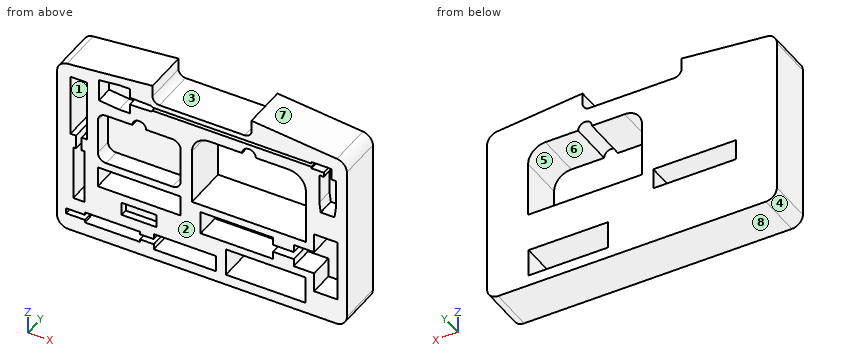
from build123d import *

# Parameters (mm, degrees)
F1_DEPTH  = 65
F11_DEPTH = 65.001
F12_DEPTH = 25.4
F13_DEPTH = 35.56
F9_W      = 120
F9_H      = 30
F8_W      = 115
F8_H      = 40
F14_DEPTH = 65.001
F15_DEPTH = 25.4
F16_DEPTH = 40.64
F10_W     = 50.8
F10_H     = 19.05
F17_DEPTH = 10.16


# Not quite as in the source:
# - a length typed as a fraction of an inch, garbled in the dataset ("3 / 203.2 mm" for 3/8 in), is restored


with BuildPart() as f1:
    # F0 (on Front) → F1 (new body)
    with BuildSketch(Plane.XZ):
        with BuildLine():
            Line((-194, -129.5), (0, -129.5))
            Line((0, -129.5), (194, -129.5))
            ThreePointArc((194, -129.5), (205.313708499, -124.813708499), (210, -113.5))
            Line((210, -113.5), (210, 115.0378975104))
            ThreePointArc((210, 115.0378975104), (205.8697706725, 125.76676251), (195.6114319773, 130.9565434007))
            Line((195.6114319773, 130.9565434007), (71.7, 143.5))
            Line((71.7, 143.5), (71.7, 126.7))
            ThreePointArc((71.7, 126.7), (68.7710678119, 119.6289321881), (61.7, 116.7))
            Line((61.7, 116.7), (0, 116.7))
            Line((0, 116.7), (-61.7, 116.7))
            ThreePointArc((-61.7, 116.7), (-68.7710678119, 119.6289321881), (-71.7, 126.7))
            Line((-71.7, 126.7), (-71.7, 143.5))
            Line((-71.7, 143.5), (-195.6114319773, 130.9565434007))
            ThreePointArc((-195.6114319773, 130.9565434007), (-205.8697706725, 125.76676251), (-210, 115.0378975104))
            Line((-210, 115.0378975104), (-210, -113.5))
            ThreePointArc((-210, -113.5), (-205.313708499, -124.813708499), (-194, -129.5))
        make_face()
    extrude(amount=F1_DEPTH)

    # F10 (on face) → F11 (cut, through all)
    with BuildSketch(Plane.XZ.offset(65)):
        with BuildLine():
            Line((-14.4175440073, -17.7396814525), (55.0347959064, -17.7396814525))
            Line((55.0347959064, -17.7396814525), (150.5824559927, -17.7396814525))
            Line((150.5824559927, -17.7396814525), (150.5824559927, 62.2603185475))
            ThreePointArc((150.5824559927, 62.2603185475), (143.2601255224, 79.9379880772), (125.5824559927, 87.2603185475))
            Line((125.5824559927, 87.2603185475), (78.0824559927, 87.2603185475))
            ThreePointArc((78.0824559927, 87.2603185475), (68.0824559927, 97.2603185475), (58.0824559927, 87.2603185475))
            Line((58.0824559927, 87.2603185475), (10.5824559927, 87.2603185475))
            ThreePointArc((10.5824559927, 87.2603185475), (-7.095213537, 79.9379880772), (-14.4175440073, 62.2603185475))
            Line((-14.4175440073, 62.2603185475), (-14.4175440073, -17.7396814525))
        make_face()
    extrude(amount=-F11_DEPTH, mode=Mode.SUBTRACT)

    # F3 (on face) → F12 (cut)
    with BuildSketch(Plane.XZ.offset(65)):
        with BuildLine():
            ThreePointArc((-151, 7.4711079597), (-147.4852813742, -1.0141734145), (-139, -4.5288920403))
            Line((-139, -4.5288920403), (-101.0147116184, -4.5288920403))
            Line((-101.0147116184, -4.5288920403), (-43, -4.5288920403))
            ThreePointArc((-43, -4.5288920403), (-34.5147186258, -1.0141734145), (-31, 7.4711079597))
            Line((-31, 7.4711079597), (-31, 58.4711079597))
            ThreePointArc((-31, 58.4711079597), (-34.5147186258, 66.956389334), (-43, 70.4711079597))
            Line((-43, 70.4711079597), (-81, 70.4711079597))
            ThreePointArc((-81, 70.4711079597), (-91, 80.4711079597), (-101, 70.4711079597))
            Line((-101, 70.4711079597), (-139, 70.4711079597))
            ThreePointArc((-139, 70.4711079597), (-147.4852813742, 66.956389334), (-151, 58.4711079597))
            Line((-151, 58.4711079597), (-151, 7.4711079597))
        make_face()
    extrude(amount=-F12_DEPTH, mode=Mode.SUBTRACT)

    # F4 (on face) → F13 (cut)
    with BuildSketch(Plane.XZ.offset(65)):
        Polygon((162.6070588827, -90.9896814525), (196.1070588827, -90.9896814525), (196.1070588827, -45.9896814525), (196.1070588827, -0.9896814525), (162.6070588827, -0.9896814525), (162.6070588827, -29.2396814525), (133.1070588827, -29.2396814525), (133.1070588827, -40.4896814525), (103.1070588827, -40.4896814525), (103.1070588827, -29.2396814525), (-1.8929411173, -29.2396814525), (-1.8929411173, -45.9896814525), (-1.8929411173, -62.7396814525), (103.1070588827, -62.7396814525), (103.1070588827, -51.4896814525), (133.1070588827, -51.4896814525), (133.1070588827, -62.7396814525), (162.6070588827, -62.7396814525), align=None)
    extrude(amount=-F13_DEPTH, mode=Mode.SUBTRACT)

    # F9 (on face) + F8 (on face) → F14 (cut, through all)
    with BuildSketch(Plane.XZ.offset(65)):
        with Locations((-91, -30.7038457692)):
            Rectangle(F9_W, F9_H)
    with BuildSketch(Plane.XZ.offset(65)):
        with Locations((92.2330532188, -93.9844995737)):
            Rectangle(F8_W, F8_H)
    extrude(amount=-F14_DEPTH, mode=Mode.SUBTRACT)

    # F7 (on face) → F15 (cut)
    with BuildSketch(Plane.XZ.offset(65)):
        Polygon((-149.4115442038, 122.7246001363), (-149.4115442038, 106.7246001363), (-149.4115442038, 90.7246001363), (-120.1630565758, 87.4952884788), (-104.6630565758, 87.4952884788), (-104.6630565758, 101.2452884788), (-73.6785290068, 102.2246001363), (-71.4424610293, 104.2246001363), (158.5575389707, 104.2246001363), (158.5575389707, 101.7246001363), (176.5575389707, 101.7246001363), (176.5575389707, 95.2246001363), (170.0575389707, 95.2246001363), (170.0575389707, 52.2246001363), (172.0575389707, 37.2246001363), (182.0575389707, 37.2246001363), (192.0575389707, 37.2246001363), (194.0575389707, 52.2246001363), (194.0575389707, 95.2246001363), (187.5575389707, 95.2246001363), (187.5575389707, 111.7246001363), (158.5575389707, 111.7246001363), (158.5575389707, 109.2246001363), (-71.4424610293, 109.2246001363), (-73.6785290068, 111.2246001363), (-104.6630565758, 112.2039117938), (-104.6630565758, 125.9539117938), (-120.1630565758, 125.9539117938), align=None)
    extrude(amount=-F15_DEPTH, mode=Mode.SUBTRACT)

    # F7 (on face) + F5 (on face) → F16 (cut)
    with BuildSketch(Plane.XZ.offset(65)):
        Polygon((-89.8567122221, -93.9844995737), (-169.8567122221, -93.9844995737), (-169.8567122221, -97.9844995737), (-196.8567122221, -97.9844995737), (-196.8567122221, -101.9844995737), (-196.8567122221, -105.9844995737), (-169.8567122221, -105.9844995737), (-169.8567122221, -109.9844995737), (-89.8567122221, -109.9844995737), (-89.8567122221, -105.9844995737), (-69.8567122221, -105.9844995737), (-69.8567122221, -113.9844995737), (20.1432877779, -113.9844995737), (20.1432877779, -101.9844995737), (20.1432877779, -89.9844995737), (-69.8567122221, -89.9844995737), (-69.8567122221, -97.9844995737), (-89.8567122221, -97.9844995737), align=None)
    with BuildSketch(Plane.XZ.offset(65)):
        Polygon((-186.5798817873, 2.1856421232), (-186.5798817873, -77.8143578768), (-178.5798817873, -77.8143578768), (-170.5798817873, -77.8143578768), (-170.5798817873, 2.1856421232), (-174.5798817873, 2.1856421232), (-174.5798817873, 22.1856421232), (-166.5798817873, 22.1856421232), (-166.5798817873, 112.1856421232), (-178.5798817873, 112.1856421232), (-190.5798817873, 112.1856421232), (-190.5798817873, 22.1856421232), (-182.5798817873, 22.1856421232), (-182.5798817873, 2.1856421232), align=None)
    extrude(amount=-F16_DEPTH, mode=Mode.SUBTRACT)

    # F10 (on face) → F17 (cut)
    with BuildSketch(Plane.XZ.offset(65)):
        with Locations((-91, -67.9338675678)):
            Rectangle(F10_W, F10_H)
    extrude(amount=-F17_DEPTH, mode=Mode.SUBTRACT)


solid = f1.part
Design review of the part built by this model. Coordinates are the model's own, in mm. Face numbers are marked on the shaded views. A direction names the side the tool comes from. Give positions to 0.01 mm unless a question says otherwise; leave off trailing zeros. Loops run counter-clockwise (first coordinate to the right, second up) from the corner with the lowest first, then second, coordinate; pieces in that order, holes last. Notation, with made-up numbers: M 86,19 L 144,19 A30 cw 144,44 Z; hole C -28,-7 d5. An arc over 180 degrees is marked long. One line per question, with ' | ' between items. Start each with the question number.
1. To check wall thickness, follow L1, parallel to X at y = -33.5, z = 48; L2, parallel to X at y = -31, z = 3; L3, parallel to X at y = -59, z = -16. State the ranges of each line that lie inside material, in increasing order.
2. Add section C-C (x = 87.5). Write out the cut boundary in (y, z).
3. Add section B-B (x = 137.5). Write out the cut boundary in (y, z).
4. For the marked faces 1, 2, 3, 4 and 5, list the 3-axis set-ups (+Z, -Z, +X, -X, +Y, -Y) from which the entire face can be reached by the end or side of a thin tool; tool diameter is ignored.
5. Insertion check: P1, Ø10, axis at x = 71.5, y = -22.5, coming from the +Z side; P2, Ø8, axis at x = -2, y = -12.5, coming from the +Z side; P3, Ø23.5, axis at x = 143, y = -50, coming from the +Z side; P4, Ø18.5, axis at y = -25.5, z = 135.5, coming from the -X side. Each pin has a flat end and moves straight along its axis. Give the tip position at first contact, or say it passes through.
6. The part is to be moulded in two halves that separate along X. For the marked faces 6, 7 and 8, say which applies: released by +X, released by -X, zero draft, split by the parting line, or undercut.
7. Add section A-A (z = -35.5). Write out the cut boundary in (x, y).
Worked out:
1) L1: x = -210 to -190.58, -166.58 to -14.42, 150.58 to 210 | L2: x = -210 to -182.58, -174.58 to -14.42, 150.58 to 210 | L3: x = -210 to -186.58, -170.58 to -151, -31 to -14.42, 150.58 to 162.61, 196.11 to 210
2) outline: M -65,-129.5 L 0,-129.5 L 0,-113.98 L -65,-113.98 Z; M -65,-73.98 L 0,-73.98 L 0,-17.74 L -65,-17.74 L -65,-29.24 L -29.44,-29.24 L -29.44,-62.74 L -65,-62.74 Z; M -65,87.26 L 0,87.26 L 0,141.9 L -65,141.9 L -65,109.22 L -39.6,109.22 L -39.6,104.22 L -65,104.22 Z
3) outline: M -65,-129.5 L 0,-129.5 L 0,-113.98 L -65,-113.98 Z; M -65,-73.98 L 0,-73.98 L 0,-17.74 L -65,-17.74 L -65,-29.24 L -29.44,-29.24 L -29.44,-62.74 L -65,-62.74 Z; M -65,84.24 L 0,84.24 L 0,136.84 L -65,136.84 L -65,109.22 L -39.6,109.22 L -39.6,104.22 L -65,104.22 Z
4) face 1: -Y | face 2: +Z, -Z, +X, -X, -Y | face 3: +Z, +Y, -Y | face 4: -Z, -X, +Y, -Y | face 5: +Y, -Y
5) P1: stops at z = 143.5 | P2: stops at z = 116.7 | P3: stops at z = 137.47 | P4: stops at x = -205.41
6) face 6: undercut | face 7: released by +X | face 8: zero draft
7) outline: M -210,-65 L -186.58,-65 L -186.58,-24.36 L -170.58,-24.36 L -170.58,-65 L -151,-65 L -151,0 L -210,0 Z; M -31,-65 L -1.89,-65 L -1.89,-29.44 L 103.11,-29.44 L 103.11,-65 L 133.11,-65 L 133.11,-29.44 L 196.11,-29.44 L 196.11,-65 L 210,-65 L 210,0 L -31,0 Z
